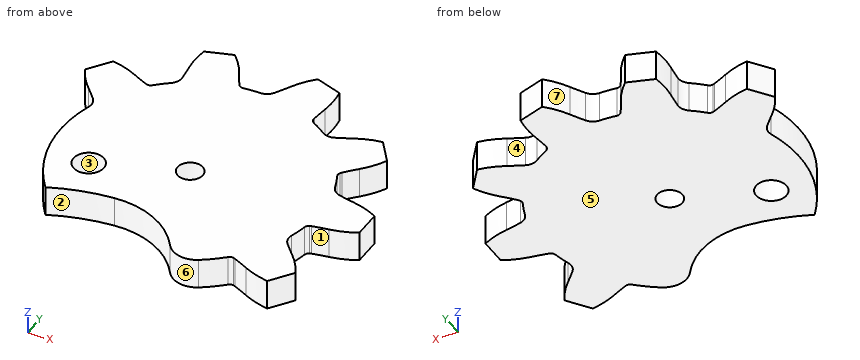
from build123d import *

# Parameters (mm, degrees)
SKETCH1_R           = 1.5
SKETCH1_R_2         = 1.25
BOSS_EXTRUDE1_DEPTH = 3


with BuildPart() as part:
    # Sketch1 → Boss-Extrude1 (new body)
    with BuildSketch(Plane.XY):
        with BuildLine():
            Line((18.079443034, -0.134472667), (18.116448206, 2.597069427))
            ThreePointArc((18.116448206, 2.597069427), (16.895577145, 3.141355734), (15.603766672, 3.48486619))
            ThreePointArc((15.603766672, 3.48486619), (14.82120671, 3.639343944), (14.043536913, 3.816807057))
            ThreePointArc((14.043536913, 3.816807057), (13.486015309, 4.11861181), (13.148996222, 4.655579763))
            ThreePointArc((13.148996222, 4.655579763), (12.877808188, 5.433093829), (12.557188118, 6.191561919))
            ThreePointArc((12.557188118, 6.191561919), (12.512759529, 6.440033201), (12.595364936, 6.678545725))
            ThreePointArc((12.595364936, 6.678545725), (12.647044724, 6.750316962), (12.70368256, 6.818243882))
            ThreePointArc((12.70368256, 6.818243882), (13.244598766, 7.404475621), (13.802549183, 7.974518889))
            ThreePointArc((13.802549183, 7.974518889), (14.673526858, 8.988509045), (15.372435088, 10.12794111))
            Line((15.372435088, 10.12794111), (13.796812742, 12.35955618))
            ThreePointArc((13.796812742, 12.35955618), (12.489183841, 12.082283047), (11.242176835, 11.600881699))
            ThreePointArc((11.242176835, 11.600881699), (10.518272782, 11.265879623), (9.784814499, 10.95234746))
            ThreePointArc((9.784814499, 10.95234746), (9.156373664, 10.868809657), (8.568097651, 11.105131008))
            ThreePointArc((8.568097651, 11.105131008), (7.891690622, 11.574752773), (7.186487179, 11.999910599))
            ThreePointArc((7.186487179, 11.999910599), (7.00449594, 12.174813619), (6.931130974, 12.416328545))
            ThreePointArc((6.931130974, 12.416328545), (6.930754726, 12.504769312), (6.936649256, 12.59301423))
            ThreePointArc((6.936649256, 12.59301423), (7.029681289, 13.385228238), (7.146009632, 14.174357956))
            ThreePointArc((7.146009632, 14.174357956), (7.254636913, 15.506641056), (7.150324186, 16.839268911))
            Line((7.150324186, 16.839268911), (4.563908504, 17.71855585))
            ThreePointArc((4.563908504, 17.71855585), (3.668991559, 16.72563219), (2.943102312, 15.603197991))
            ThreePointArc((2.943102312, 15.603197991), (2.55436091, 14.906675492), (2.145270277, 14.221906682))
            ThreePointArc((2.145270277, 14.221906682), (1.685953249, 13.784934925), (1.071121753, 13.630342949))
            ThreePointArc((1.071121753, 13.630342949), (0.247860223, 13.612692862), (-0.572562847, 13.542144585))
            ThreePointArc((-0.572562847, 13.542144585), (-0.822602268, 13.576672334), (-1.023914683, 13.728939169))
            ThreePointArc((-1.023914683, 13.728939169), (-1.076203253, 13.8002681), (-1.12330354, 13.875124455))
            ThreePointArc((-1.12330354, 13.875124455), (-1.513690755, 14.570721908), (-1.883417958, 15.277517345))
            ThreePointArc((-1.883417958, 15.277517345), (-2.578633, 16.419206529), (-3.446322769, 17.436011628))
            Line((-3.446322769, 17.436011628), (-6.055608905, 16.62711271))
            ThreePointArc((-6.055608905, 16.62711271), (-6.195986038, 15.297801614), (-6.123492507, 13.963066277))
            ThreePointArc((-6.123492507, 13.963066277), (-6.028585255, 13.171071275), (-5.957049521, 12.376624229))
            ThreePointArc((-5.957049521, 12.376624229), (-6.071799248, 11.753126877), (-6.478341494, 11.266670455))
            ThreePointArc((-6.478341494, 11.266670455), (-7.133999602, 10.768490249), (-7.756268571, 10.229182913))
            ThreePointArc((-7.756268571, 10.229182913), (-7.978849614, 10.110146965), (-8.231214979, 10.115004953))
            ThreePointArc((-8.231214979, 10.115004953), (-8.315443414, 10.14197682), (-8.397547808, 10.17485203))
            ThreePointArc((-8.397547808, 10.17485203), (-9.122239624, 10.508138343), (-9.836799148, 10.862627665))
            ThreePointArc((-9.836799148, 10.862627665), (-11.070307997, 11.377636469), (-12.369946808, 11.690233824))
            Line((-12.369946808, 11.690233824), (-14.005444781, 9.502120943))
            ThreePointArc((-14.005444781, 9.502120943), (-13.337662809, 8.344174067), (-12.494476564, 7.306961125))
            ThreePointArc((-12.494476564, 7.306961125), (-11.952172002, 6.722008792), (-11.427334121, 6.12133528))
            ThreePointArc((-11.427334121, 6.12133528), (-11.153686052, 5.549467129), (-11.196653727, 4.91695608))
            ThreePointArc((-11.196653727, 4.91695608), (-11.678838592, -1.351524146), (-9.118252224, -7.093452745))
            ThreePointArc((-9.118252224, -7.093452745), (-6.159667353, -6.136962556), (-3.085467527, -5.670707959))
            ThreePointArc((-3.085467527, -5.670707959), (1.133419318, -6.513694494), (4.3378838, -9.384415639))
            ThreePointArc((4.3378838, -9.384415639), (5.797671296, -10.408859622), (7.558678835, -10.127226075))
            ThreePointArc((7.558678835, -10.127226075), (8.631472289, -9.400453805), (9.623684759, -8.567028257))
            ThreePointArc((9.623684759, -8.567028257), (9.846265801, -8.447992309), (10.098631166, -8.452850297))
            ThreePointArc((10.098631166, -8.452850297), (10.182859602, -8.479822164), (10.264963995, -8.512697373))
            ThreePointArc((10.264963995, -8.512697373), (10.989655811, -8.845983686), (11.704215336, -9.200473008))
            ThreePointArc((11.704215336, -9.200473008), (12.937724185, -9.715481811), (14.237362996, -10.028079165))
            Line((14.237362996, -10.028079165), (15.872860968, -7.839966284))
            ThreePointArc((15.872860968, -7.839966284), (15.205078995, -6.682019407), (14.361892749, -5.644806466))
            ThreePointArc((14.361892749, -5.644806466), (13.819588187, -5.059854134), (13.294750306, -4.459180622))
            ThreePointArc((13.294750306, -4.459180622), (13.021102236, -3.887312471), (13.064069415, -3.254802895))
            ThreePointArc((13.064069415, -3.254802895), (13.301685284, -2.466379753), (13.488114756, -1.664309679))
            ThreePointArc((13.488114756, -1.664309679), (13.598219027, -1.43717772), (13.80524235, -1.292771275))
            ThreePointArc((13.80524235, -1.292771275), (13.889238251, -1.265083742), (13.974985665, -1.243420593))
            ThreePointArc((13.974985665, -1.243420593), (14.757174439, -1.087091722), (15.543628834, -0.953872058))
            ThreePointArc((15.543628834, -0.953872058), (16.844273034, -0.645484622), (18.079443034, -0.134472667))
        make_face()
        with Locations((-7.418095669, -2.256802895)):
            Circle(SKETCH1_R, mode=Mode.SUBTRACT)
        with Locations((0.933711072, 0.831073783)):
            Circle(SKETCH1_R_2, mode=Mode.SUBTRACT)
    extrude(amount=BOSS_EXTRUDE1_DEPTH)


solid = part.part
Work out the finished part from the listing and answer in its coordinate system (mm). Face numbers are marked on the shaded views. A direction names the side the tool comes from. Round coordinates to 2 decimals unless told otherwise and drop trailing zeros. Loops run counter-clockwise (first coordinate to the right, second up) from the corner with the lowest first, then second, coordinate; pieces in that order, holes last. Notation, with made-up numbers: (-19.75, 67) -> (-11.75, 67) arc R21 cw to (-11.75, 87) -> close; hole circle Ø4 at (19.25, 36). An arc over 180 degrees is marked (long way). Use one line per item in the form item = value.
(1) A tool of negligible diameter and unlimited length cuts with its end or side. For the marked faces 1, 2, 3 and 4, from which of +Z, -Z, +X, -X, +Y, -Y can it reach the whole face along a straight path? Write none if from no direction.
Answer list:
face_1 = +Z, -Z, +X
face_2 = +Z, -Z, -Y
face_3 = +Z, -Z
face_4 = +Z, -Z, +Y
(2) Straight lines are drawn through the part: line 1 (Y direction, x = -7, z = 2.6); line 2 (Y direction, x = 14, z = 2.85); line 3 (X direction, y = 15.75, z = 1.3). For each, find the intervals that lie inside material, in ascending order.
Answer list:
line_1 = -6.36 to -3.7, -0.82 to 10.88
line_2 = -9.99 to -5.26, -1.24 to 3.83, 8.18 to 12.07
line_3 = -6.17 to -2.14, 3.02 to 7.25
(3) Find section B-B on z = 2.3. Give the number of separate pieces and of enclosed holes in the cut face, then the cut area to 3 significant figures.
Answer list:
separate_pieces = 1
enclosed_holes = 2
area = 555 mm2
(4) For a pull along X with two mould halves and no side action, classify the marked faces 5, 6 and 7 as released by +X, released by -X, zero draft, split by the parting line, or undercut.
Answer list:
face_5 = zero draft
face_6 = split by the parting line
face_7 = undercut
(5) Flat-ended cylindrical pins translate along their axes: P1, Ø1.5, axis at x = -10.5, z = 2, coming from the -Y side; P2, Ø2, axis at x = 0.93, y = 0.83, coming from the +Z side; P3, Ø1.5, axis at y = 7.5, z = 1, coming from the -X side. Find the tip coordinate at first contact, or state that the pin passes through.
Answer list:
P1 = -6.22
P2 = through
P3 = -13.27
(6) Find section C-C on x = -5.5. Give the vertices of the cut face in (y, z), then the cut area to 3 significant figures.
Answer list:
outline = (-5.99, 0) -> (16.8, 0) -> (16.8, 3) -> (-5.99, 3) -> close
area = 68.4 mm2
(7) Find section D-D on x = 6. Give the vertices of the cut face in (y, z).
Answer list:
outline = (-10.45, 0) -> (17.23, 0) -> (17.23, 3) -> (-10.45, 3) -> close
(8) Find section A-A on x = 1.5. Give the vertices of the cut face in (y, z).
Answer list:
outline = (-6.71, 0) -> (-0.28, 0) -> (-0.28, 3) -> (-6.71, 3) -> close; (1.95, 0) -> (13.7, 0) -> (13.7, 3) -> (1.95, 3) -> close
